Build history of the part. All positions in model axes, mm. A direction names the side the tool comes from. Give positions to 0.01 mm unless a question says otherwise; leave off trailing zeros. Order: outer loops, then holes, each group sorted by start corner. A loop starts at its lowest first (then second) coordinate and runs counter-clockwise, first axis right, second up. Notation, with made-up numbers: (33, -33.75) - (66, -33.75) arc R21 ccw to (66, -29.75) - close; hole circle Ø8 at (3, 23). An arc over 180 degrees is marked (long way). Answer in a Markdown table with one row per item.
```python
from build123d import *

# Parameters (mm, degrees)
SKICA1_W                 = 75
SKICA1_H                 = 45
P_IDAT_VYSUNUT_M1_DEPTH  = 13
SKICA2_W                 = 71
SKICA2_H                 = 41
ODEBRAT_VYSUNUT_M1_DEPTH = 12
ZAOBLIT1_R               = 2
ZKOSEN_2_SIZE            = 0.5
SKICA3_W                 = 50
SKICA3_H                 = 38.5
ODEBRAT_VYSUNUT_M2_DEPTH = 6
SKICA4_W                 = 7.3
SKICA4_H                 = 7.3
P_IDAT_VYSUNUT_M2_DEPTH  = 4.22
ZAOBLIT2_R               = 1
SKICA6_W                 = 92.209043038
SKICA6_H                 = 16.914138174
ODEBRAT_VYSUNUT_M3_DEPTH = 64.22
SKICA5_W                 = 5.279513812
SKICA5_H                 = 9.3
ODEBRAT_VYSUNUT_M4_DEPTH = 6.2
SKICA7_W                 = 4
SKICA7_H                 = 7.314220015
ODEBRAT_VYSUNUT_M5_DEPTH = 1.9
SKICA8_W                 = 14.8
SKICA8_H                 = 7.292326558
ODEBRAT_VYSUNUT_M6_DEPTH = 1.9
SKICA9_R                 = 1.125
ODEBRAT_VYSUNUT_M7_DEPTH = 3


with BuildPart() as part:
    # Skica1 → Přidat vysunutím1 (new body)
    with BuildSketch(Plane.XY):
        Rectangle(SKICA1_W, SKICA1_H)
    extrude(amount=P_IDAT_VYSUNUT_M1_DEPTH)

    # Skica2 → Odebrat vysunutím1 (cut)
    with BuildSketch(Plane.XY.offset(13)):
        Rectangle(SKICA2_W, SKICA2_H)
    extrude(amount=-ODEBRAT_VYSUNUT_M1_DEPTH, mode=Mode.SUBTRACT)

    # Zaoblit1
    zaoblit1_edges = [part.edges().sort_by_distance(p)[0] for p in [
        (35.5, 20.5, 7),
        (35.5, -20.5, 7),
        (-35.5, -20.5, 7),
        (-35.5, 20.5, 7),
        (37.5, -22.5, 6.5),
        (-37.5, -22.5, 6.5),
        (-37.5, 22.5, 6.5),
        (37.5, 22.5, 6.5),
    ]]
    fillet(zaoblit1_edges, radius=ZAOBLIT1_R)

    # Zkosení2
    zkosen_2_edges = [part.edges().sort_by_distance(p)[0] for p in [
        (0, 22.5, 0),
        (37.5, 0, 0),
        (0, -22.5, 0),
        (-37.5, 0, 0),
        (-36.914213562, 21.914213562, 0),
        (-36.914213562, -21.914213562, 0),
        (36.914213562, -21.914213562, 0),
        (36.914213562, 21.914213562, 0),
    ]]
    chamfer(zkosen_2_edges, length=ZKOSEN_2_SIZE)

    # Skica3 → Odebrat vysunutím2 (cut, symmetric)
    with BuildSketch(Plane(origin=(0, 0, 0), x_dir=(-1, 0, 0), z_dir=(0, 0, -1))):
        with Locations((3, 0)):
            Rectangle(SKICA3_W, SKICA3_H)
    extrude(amount=ODEBRAT_VYSUNUT_M2_DEPTH, both=True, mode=Mode.SUBTRACT)

    # Skica4 → Přidat vysunutím2 (add)
    with BuildSketch(Plane.XY.offset(1)):
        with Locations((-33.264213562, 18.264213562)):
            Rectangle(SKICA4_W, SKICA4_H)
        with Locations((-33.264213562, -18.264213562)):
            Rectangle(SKICA4_W, SKICA4_H)
        with Locations((33.264213562, -18.264213562)):
            Rectangle(SKICA4_W, SKICA4_H)
        with Locations((33.264213562, 18.264213562)):
            Rectangle(SKICA4_W, SKICA4_H)
    extrude(amount=P_IDAT_VYSUNUT_M2_DEPTH)

    # Zaoblit2
    zaoblit2_edges = [part.edges().sort_by_distance(p)[0] for p in [
        (-29.614213562, 14.614213562, 3.11),
        (-29.614213562, -14.614213562, 3.11),
        (29.614213562, -14.614213562, 3.11),
        (29.614213562, 14.614213562, 3.11),
    ]]
    fillet(zaoblit2_edges, radius=ZAOBLIT2_R)

    # Skica6 → Odebrat vysunutím3 (cut)
    with BuildSketch(Plane.XZ.offset(22.5)):
        with Locations((-2.449143373, 16.957069087)):
            Rectangle(SKICA6_W, SKICA6_H)
    extrude(amount=-ODEBRAT_VYSUNUT_M3_DEPTH, mode=Mode.SUBTRACT)

    # Skica5 → Odebrat vysunutím4 (cut)
    with BuildSketch(Plane.XY.offset(13)):
        with Locations((36.7595999, 2.55)):
            Rectangle(SKICA5_W, SKICA5_H)
    extrude(amount=-ODEBRAT_VYSUNUT_M4_DEPTH, mode=Mode.SUBTRACT)

    # Skica7 → Odebrat vysunutím5 (cut)
    with BuildSketch(Plane.XY.offset(8.5)):
        with Locations((-14.5, 18.092889993)):
            Rectangle(SKICA7_W, SKICA7_H)
    extrude(amount=-ODEBRAT_VYSUNUT_M5_DEPTH, mode=Mode.SUBTRACT)

    # Skica8 → Odebrat vysunutím6 (cut)
    with BuildSketch(Plane.XY.offset(8.5)):
        with Locations((0.1, 20.570563513)):
            Rectangle(SKICA8_W, SKICA8_H)
    extrude(amount=-ODEBRAT_VYSUNUT_M6_DEPTH, mode=Mode.SUBTRACT)

    # Skica9 → Odebrat vysunutím7 (cut)
    with BuildSketch(Plane.XY.offset(5.22)):
        with Locations((-31.914213562, 16.914213562)):
            Circle(SKICA9_R)
        with Locations((-31.914213562, -16.914213562)):
            Circle(SKICA9_R)
        with Locations((32.114213562, -16.914213562)):
            Circle(SKICA9_R)
        with Locations((32.114213562, 16.914213562)):
            Circle(SKICA9_R)
    extrude(amount=-ODEBRAT_VYSUNUT_M7_DEPTH, mode=Mode.SUBTRACT)


solid = part.part
```
1. Two-plate mould, pull along Y, no slides. Class faces 1 (the face through (-34.9, 19.93, 6.84)), 2 (the face through (36.65, 21.67, 0.14)), 3 (the face through (37.5, 0, 4)): +Y half, -Y half, draft (parallel to the pull), parting line (faces both ways), or undercut.
Check result:
| item | result |
|---|---|
| face 1 | undercut |
| face 2 | +Y half |
| face 3 | draft |
2. Drop flat-ended pins along their axis: P1, Ø0.7, axis at x = 31.5, y = -16.5, coming from the +Z side; P2, Ø2.5, axis at x = 32.11, y = -16.91, coming from the +Z side; P3, Ø8, axis at x = 25, y = -8.5, coming from the +Z side. Give the stop position or say it passes through.
Check result:
| item | result |
|---|---|
| P1 | stops at z = 2.22 |
| P2 | stops at z = 5.22 |
| P3 | stops at z = 1 |
3. Cut at C-C on z = 3.25. Write the cut outline in (x, y) (3 decimals).
Check result:
| item | result |
|---|---|
| outline | (-37.5, -20.5) arc R2 ccw to (-35.5, -22.5) - (35.5, -22.5) arc R2 ccw to (37.5, -20.5) - (37.5, 20.5) arc R2 ccw to (35.5, 22.5) - (-35.5, 22.5) arc R2 ccw to (-37.5, 20.5) - close; hole (-35.5, -14.614) - (-30.614, -14.614) arc R1 cw to (-29.614, -15.614) - (-29.614, -20.5) - (29.614, -20.5) - (29.614, -15.614) arc R1 cw to (30.614, -14.614) - (35.5, -14.614) - (35.5, 14.614) - (30.614, 14.614) arc R1 cw to (29.614, 15.614) - (29.614, 20.5) - (-29.614, 20.5) - (-29.614, 15.614) arc R1 cw to (-30.614, 14.614) - (-35.5, 14.614) - close; hole circle Ø2.25 at (-31.914, -16.914); hole circle Ø2.25 at (-31.914, 16.914); hole circle Ø2.25 at (32.114, -16.914); hole circle Ø2.25 at (32.114, 16.914) |
4. Probe line 1 (Y direction, x = 1.5, z = 2.5); line 2 (X direction, y = 0, z = 0.5); line 3 (X direction, y = 11, z = 2.5). List the from-to ranges inside material, lowest first.
Check result:
| item | result |
|---|---|
| line 1 | y = -22.5 to -20.5, 20.5 to 22.5 |
| line 2 | x = -37.5 to -28, 22 to 37.5 |
| line 3 | x = -37.5 to -35.5, 35.5 to 37.5 |
5. Cut at B-B on x = -19.5. Write the cut outline in (y, z).
Check result:
| item | result |
|---|---|
| outline | (-22.5, 0.5) - (-22, 0) - (-19.25, 0) - (-19.25, 1) - (-20.5, 1) - (-20.5, 8.5) - (-22.5, 8.5) - close; (19.25, 0) - (22, 0) - (22.5, 0.5) - (22.5, 8.5) - (20.5, 8.5) - (20.5, 1) - (19.25, 1) - close |
6. Which spindle directions (+Z, -Z, +X, -X, +Y, -Y) get a long thin tool onto all of the face, cutting with end or side? Do faces 4 (the face through (29.614, -18, 3)), 5 (the face through (36, -2.1, 8)), 6 (the face through (-36.67, 21.65, 0.14)). Say none if no direction does.
Check result:
| item | result |
|---|---|
| face 4 | +Z |
| face 5 | +Z, +X |
| face 6 | -Z, -X, +Y |
7. Cut at A-A on y = 1. Write the cut outline in (x, z).
Check result:
| item | result |
|---|---|
| outline | (-37.5, 0.5) - (-37, 0) - (-28, 0) - (-28, 1) - (-35.5, 1) - (-35.5, 8.5) - (-37.5, 8.5) - close; (22, 0) - (37, 0) - (37.5, 0.5) - (37.5, 6.8) - (35.5, 6.8) - (35.5, 1) - (22, 1) - close |
